Here's how the part is built. I have some questions about the finished solid (model axes, mm). Round coordinates to 2 decimals unless told otherwise and drop trailing zeros. Order: outer loops, then holes, each group sorted by start corner. A loop starts at its lowest first (then second) coordinate and runs counter-clockwise, first axis right, second up.
```python
from build123d import *

# Parameters (mm, degrees)
SKETCH1_W                   = 165.1
SKETCH1_H                   = 38.1
BOSS_EXTRUDE1_DEPTH         = 3.175
F_1_4_0_25_DIAMETER_HOLE1_D = 7.9375
SKETCH4_W                   = 50.8
SKETCH4_H                   = 355.6
SKETCH4_R                   = 4.7625
BOSS_EXTRUDE2_DEPTH         = 6.35
CUT_EXTRUDE1_REACH          = 272.08
SKETCH5_W                   = 38.1
SKETCH5_H                   = 60.325


with BuildPart() as part:
    # Sketch1 → Boss-Extrude1 (new, symmetric)
    with BuildSketch(Plane(origin=(0, 0, 0), x_dir=(1, 0, 0), z_dir=(0, 1, 0))):
        Polygon((0, 0), (0, -177.8), (38.1, -177.8), (38.1, -38.1), (38.1, 0), align=None)
        with Locations((120.65, -19.05)):
            Rectangle(SKETCH1_W, SKETCH1_H)
        with Locations((120.65, 19.05)):
            Rectangle(SKETCH1_W, SKETCH1_H)
        Polygon((0, 177.8), (0, 0), (38.1, 0), (38.1, 38.1), (38.1, 177.8), align=None)
    extrude(amount=BOSS_EXTRUDE1_DEPTH, both=True)

    # 1/4 (0.25) Diameter Hole1 (through all)
    with Locations(Plane(origin=(0, 3.175, 0), x_dir=(1, 0, 0), z_dir=(0, 1, 0))):
        with Locations((190.5, 25.4), (190.5, -25.4)):
            Hole(F_1_4_0_25_DIAMETER_HOLE1_D / 2)

    # Sketch4 → Boss-Extrude2 (add)
    with BuildSketch(Plane.XZ.offset(3.175)):
        with Locations((-25.4, 0)):
            Rectangle(SKETCH4_W, SKETCH4_H)
        with Locations(Location((-38.1, -165.1, 0), (0, 0, 270))):
            Circle(SKETCH4_R, mode=Mode.SUBTRACT)
        with Locations(Location((-38.1, 165.1, 0), (0, 0, 270))):
            Circle(SKETCH4_R, mode=Mode.SUBTRACT)
    extrude(amount=-BOSS_EXTRUDE2_DEPTH)

    # Sketch5 → Cut-Extrude1 (cut, up to next)
    with BuildSketch(Plane.XZ.offset(3.175), mode=Mode.PRIVATE) as cut_extrude1_sk1:
        with Locations((19.05, 147.6375)):
            Rectangle(SKETCH5_W, SKETCH5_H)
    cut_extrude1_tool1 = extrude(cut_extrude1_sk1.sketch, amount=-CUT_EXTRUDE1_REACH, mode=Mode.PRIVATE) & part.part
    # Sketch5 → Cut-Extrude1 (cut, up to next)
    with BuildSketch(Plane.XZ.offset(3.175), mode=Mode.PRIVATE) as cut_extrude1_sk2:
        with Locations((19.05, -147.6375)):
            Rectangle(SKETCH5_W, SKETCH5_H)
    cut_extrude1_tool2 = extrude(cut_extrude1_sk2.sketch, amount=-CUT_EXTRUDE1_REACH, mode=Mode.PRIVATE) & part.part
    add(cut_extrude1_tool1.solids().sort_by_distance((19.05, -3.175, 147.6375))[0], mode=Mode.SUBTRACT)
    add(cut_extrude1_tool2.solids().sort_by_distance((19.05, -3.175, -147.6375))[0], mode=Mode.SUBTRACT)


solid = part.part
```
1. I'm going to push flat-ended pins straight in: P1, Ø3, axis at x = 131, y = 1, coming from the +Z side; P2, Ø1.9, axis at x = 131.5, y = 1, coming from the -Z side; P3, Ø7.5, axis at x = -38.1, z = -165.1, coming from the -Y side; P4, Ø3, axis at y = -1, z = -149, coming from the +X side. Where does each tip first touch, or does it pass through?
Evaluation:
P1: stops at z = 38.1
P2: stops at z = -38.1
P3: passes through
P4: stops at x = 0
2. If we section it at D-D, the plane x = -38.1: Write out the boundary of the cut face in (y, z) (1 decimal).
Evaluation:
outline: (-3.2, -177.8) - (3.2, -177.8) - (3.2, -169.9) - (-3.2, -169.9) - close; (-3.2, -160.3) - (3.2, -160.3) - (3.2, 160.3) - (-3.2, 160.3) - close; (-3.2, 169.9) - (3.2, 169.9) - (3.2, 177.8) - (-3.2, 177.8) - close
3. If we mould it in two halves opening along Z, with no side actions, what happens to faces 1 (the cylindrical face through (186.834, -0.044, -23.88)), 2 (the flat face through (18, 3.175, 2))? For each: released by +Z, released by -Z, zero draft, split by the parting line, or undercut.
Evaluation:
face 1: undercut
face 2: zero draft
4. If we section it at C-C, the plane y = 2: Write out the boundary of the cut face in (x, z) (1 decimal).
Evaluation:
outline: (-50.8, -177.8) - (0, -177.8) - (0, -117.5) - (38.1, -117.5) - (38.1, -38.1) - (203.2, -38.1) - (203.2, 38.1) - (38.1, 38.1) - (38.1, 117.5) - (0, 117.5) - (0, 177.8) - (-50.8, 177.8) - close; hole circle Ø9.5 at (-38.1, -165.1); hole circle Ø9.5 at (-38.1, 165.1); hole circle Ø7.9 at (190.5, -25.4); hole circle Ø7.9 at (190.5, 25.4)
5. I need wall thicknesses on probe 1 along Z at (x, y) = (190.5, 1.5); probe 2 along Z at (x, y) = (191.5, 3); probe 3 along X at (y, z) = (-0.75, -25.4). Which ranges of each line are inside material? Lowest first, please.
Evaluation:
probe 1: z = -38.1 to -29.37, -21.43 to 21.43, 29.37 to 38.1
probe 2: z = -38.1 to -29.24, -21.56 to 21.56, 29.24 to 38.1
probe 3: x = -50.8 to 186.53, 194.47 to 203.2
6. If we section it at A-A, the plane x = 190.5: Write out the boundary of the cut face in (y, z) (3 decimals).
Evaluation:
outline: (-3.175, -38.1) - (3.175, -38.1) - (3.175, -29.369) - (-3.175, -29.369) - close; (-3.175, -21.431) - (3.175, -21.431) - (3.175, 21.431) - (-3.175, 21.431) - close; (-3.175, 29.369) - (3.175, 29.369) - (3.175, 38.1) - (-3.175, 38.1) - close
7. If we section it at B-B, the plane z = 25.4: Write out the boundary of the cut face in (x, y) (3 decimals), and give its area (3 significant figures).
Evaluation:
outline: (-50.8, -3.175) - (186.531, -3.175) - (186.531, 3.175) - (-50.8, 3.175) - close; (194.469, -3.175) - (203.2, -3.175) - (203.2, 3.175) - (194.469, 3.175) - close
area: 1,560 mm2
